Could you check a few things on this model? Use its own coordinates, in mm. A direction names the side the tool comes from. Coordinates: 2 decimals unless noted, no trailing zeros. Order: outer loops, then holes, each group sorted by start corner. A loop starts at its lowest first (then second) coordinate and runs counter-clockwise, first axis right, second up. Notation, with made-up numbers: (45, 14.25) - (67, 14.25) arc R8 ccw to (67, 29.25) - close; hole circle Ø2 at (70, 64.5). An arc over 180 degrees is marked (long way). Answer as a JSON object with one key per item and string values. Group by question number.
(1) Please list where these lines run through material, in increasing order: probe 1 along Y at (x, z) = (-6.5, 3.75); probe 2 along X at (y, z) = (-3.5, 12); probe 3 along X at (y, z) = (1, 12).
(2) Which directions (+Z, -Z, +X, -X, +Y, -Y) give clear straight access to the entire face, cutting with the end or side of a thin tool? Please do faces 5 (the conical face through (-21.01, 0.2, 14.16)), 6 (the conical face through (48.42, 0.312, 14.826)), 7 (the cylindrical face through (-20.85, 0.2, 6.9)).
(3) Will these pins go through, and if not, where does the flat tip stop? P1, Ø1.5, axis at y = -12, z = 10, coming from the -X side; P2, Ø1.5, axis at y = 5, z = 7.5, coming from the +X side; P3, Ø5, axis at y = -6.5, z = 12, coming from the +X side.
(4) Imagine slicing it at A-A, the plane x = 9.5. Write out the boundary of the cut face in (y, z), and give its area (3 significant figures).
(5) Imagine slicing it at C-C, the plane y = 0. Write out the boundary of the cut face in (x, z), and give its area (3 significant figures).
(6) We'd pull the mould along X, two halves only. Please class faces 1 (the conical face through (21.01, -0.2, 14.16)), 2 (the cylindrical face through (-49.246, 0.33, 6.902)), 3 (the cylindrical face through (49.246, -0.33, 6.902)), 4 (the flat face through (-1, -12, 15)): pulls with the +X half, pulls with the -X half, needs draft (parallel to the pull), parting line crosses it, or undercut.
(7) Imagine slicing it at B-B, the plane z = 6.75. Write out the boundary of the cut face in (x, y), and give its area (3 significant figures).
from build123d import *

# Parameters (mm, degrees)
SKETCH_R        = 5
PAD_DEPTH       = 15
CHAMFER_SIZE    = 1
CHAMFER001_SIZE = 1
CHAMFER002_SIZE = 1


with BuildPart() as part:
    # Sketch → Pad (new body)
    with BuildSketch(Plane.XY):
        with BuildLine():
            ThreePointArc((-34.25, 15), (-49.25, 0), (-34.25, -15))
            Line((-34.25, -15), (34.25, -15))
            ThreePointArc((34.25, -15), (49.25, 0), (34.25, 15))
            Line((-34.25, 15), (34.25, 15))
        make_face()
        with Locations((-34.25, 0)):
            Circle(SKETCH_R, mode=Mode.SUBTRACT)
        with Locations((34.25, 0)):
            Circle(SKETCH_R, mode=Mode.SUBTRACT)
        with BuildLine():
            ThreePointArc((-11.85289, 9), (-20.85289, 0), (-11.85289, -9))
            Line((-11.85289, -9), (11.85289, -9))
            ThreePointArc((11.85289, -9), (20.85289, 0), (11.85289, 9))
            Line((-11.85289, 9), (11.85289, 9))
        make_face(mode=Mode.SUBTRACT)
    extrude(amount=PAD_DEPTH)

    # Chamfer
    chamfer_edges = [part.edges().sort_by_distance(p)[0] for p in [
        (-39.25, 0, 15),
        (29.25, 0, 15),
    ]]
    chamfer(chamfer_edges, length=CHAMFER_SIZE)

    # Chamfer001
    chamfer001_edges = [part.edges().sort_by_distance(p)[0] for p in [
        (0, 15, 15),
        (49.25, 0, 15),
        (0, -15, 15),
        (-49.25, 0, 15),
    ]]
    chamfer(chamfer001_edges, length=CHAMFER001_SIZE)

    # Chamfer002
    chamfer002_edges = [part.edges().sort_by_distance(p)[0] for p in [
        (20.85289, 0, 15),
        (0, -9, 15),
        (-20.85289, 0, 15),
        (0, 9, 15),
    ]]
    chamfer(chamfer002_edges, length=CHAMFER002_SIZE)


solid = part.part
Result set:
{
 "1": {"probe 1": "y = -15 to -9, 9 to 15", "probe 2": "x = -48.84 to -37.82, -30.68 to -20.14, 20.14 to 30.68, 37.82 to 48.84", "probe 3": "x = -49.22 to -39.15, -29.35 to -20.8, 20.8 to 29.35, 39.15 to 49.22"},
 "2": {"face 5": "+Z", "face 6": "+Z, +X", "face 7": "+Z, -Z"},
 "3": {"P1": "stops at x = -44.17", "P2": "stops at x = 48.64", "P3": "stops at x = 48.71"},
 "4": {"outline": "(-15, 0) - (-9, 0) - (-9, 14) - (-10, 15) - (-14, 15) - (-15, 14) - close; (9, 0) - (15, 0) - (15, 14) - (14, 15) - (10, 15) - (9, 14) - close", "area": "178 mm^2"},
 "5": {"outline": "(-49.25, 0) - (-39.25, 0) - (-39.25, 14) - (-40.25, 15) - (-48.25, 15) - (-49.25, 14) - close; (-29.25, 0) - (-20.85, 0) - (-20.85, 14) - (-21.85, 15) - (-28.25, 15) - (-29.25, 14) - close; (20.85, 0) - (29.25, 0) - (29.25, 14) - (28.25, 15) - (21.85, 15) - (20.85, 14) - close; (39.25, 0) - (49.25, 0) - (49.25, 14) - (48.25, 15) - (40.25, 15) - (39.25, 14) - close", "area": "548 mm^2"},
 "6": {"face 1": "undercut", "face 2": "pulls with the -X half", "face 3": "pulls with the +X half", "face 4": "needs draft"},
 "7": {"outline": "(-34.25, -15) - (34.25, -15) arc R15 ccw to (34.25, 15) - (-34.25, 15) arc R15 ccw to start; hole circle Ø10 at (-34.25, 0); hole (-11.85, -9) - (11.85, -9) arc R9 ccw to (11.85, 9) - (-11.85, 9) arc R9 ccw to start; hole circle Ø10 at (34.25, 0)", "area": "1,920 mm^2"}
}
